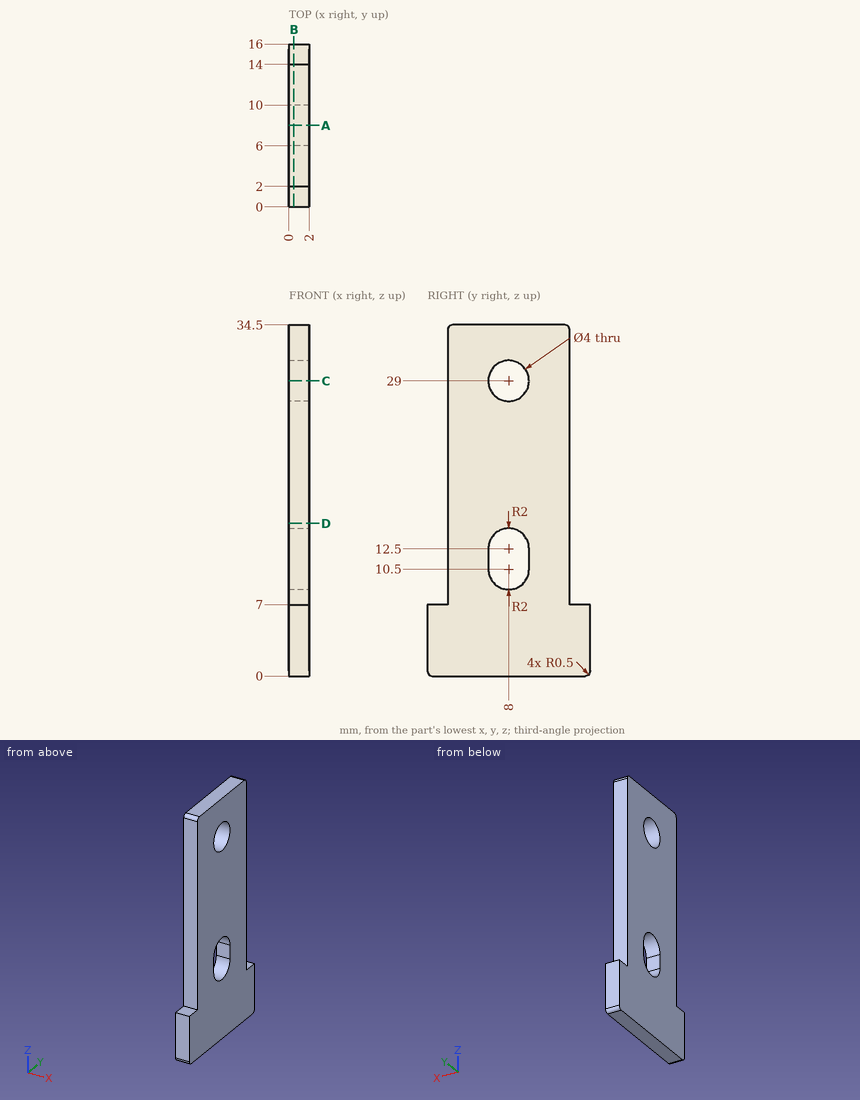
Verification items for this drawing (mm, ordinates from the low corner). Give positions to 0.01 mm unless a question says otherwise; leave off trailing zeros. Loops run counter-clockwise (first coordinate to the right, second up) from the corner with the lowest first, then second, coordinate; pieces in that order, holes last.
(1) Section check B-B on x = 0.5. Record the cut outline in (y, z), then the cut area to 3 significant figures.
From the geometry:
outline: (0, 0.5) arc R0.5 ccw to (0.5, 0) - (15.5, 0) arc R0.5 ccw to (16, 0.5) - (16, 7) - (14, 7) - (14, 34) arc R0.5 ccw to (13.5, 34.5) - (2.5, 34.5) arc R0.5 ccw to (2, 34) - (2, 7) - (0, 7) - close; hole (6, 10.5) arc R2 ccw to (10, 10.5) - (10, 12.5) arc R2 ccw to (6, 12.5) - close; hole circle Ø4 at (8, 29)
area: 409 mm2
(2) Section check D-D on z = 15. Record the cut outline in (x, y), then the cut area to 3 significant figures.
From the geometry:
outline: (0, 2) - (2, 2) - (2, 14) - (0, 14) - close
area: 24.0 mm2
(3) Thickness scan on L1, parallel to Y at x = 1.1, z = 29; L2, parallel to Z at x = 1.15, y = 7.75; L3, parallel to Y at x = 1.8, z = 15. Record the ranges inside material, lowest first.
From the geometry:
L1: y = 2 to 6, 10 to 14
L2: z = 0 to 8.52, 14.48 to 27.02, 30.98 to 34.5
L3: y = 2 to 14
(4) Depth check by flat-ended pin: pin 1 Ø1 at (x, z) = (1.5, 25) entering from +Y; pin 2 Ø0.6 at (x, y) = (1, 15) entering from +Z. Enter the tip coordinate at first touch or a pass-through.
From the geometry:
pin 1: stops at y = 14
pin 2: stops at z = 7
(5) Section check C-C on z = 29. Record the cut outline in (x, y), then the cut area to 3 significant figures.
From the geometry:
outline: (0, 2) - (2, 2) - (2, 6) - (0, 6) - close; (0, 10) - (2, 10) - (2, 14) - (0, 14) - close
area: 16.0 mm2
(6) Section check A-A on y = 8. Record the cut outline in (x, z), then the cut area to 3 significant figures.
From the geometry:
outline: (0, 0) - (2, 0) - (2, 8.5) - (0, 8.5) - close; (0, 14.5) - (2, 14.5) - (2, 27) - (0, 27) - close; (0, 31) - (2, 31) - (2, 34.5) - (0, 34.5) - close
area: 49.0 mm2
